Check sheet for the drawn part. Datum: minimum x, y, z corner. Units: mm. A direction names the side the tool comes from. Give positions to 0.01 mm unless a question says otherwise; leave off trailing zeros. Loops run counter-clockwise (first coordinate to the right, second up) from the corner with the lowest first, then second, coordinate; pieces in that order, holes last. Notation, with made-up numbers: (55, 76) - (111, 76) arc R5 ccw to (111, 81) - close; hole circle Ø11 at (3.5, 62.25). An arc over 180 degrees is marked (long way). One line per item, written item: value. Start each with the question number.
1. Sectioned sample at D-D (x = 14). Record the cut outline in (y, z), plus the area to 3 significant figures.
2. Scan lines: L1, parallel to X at y = 27, z = 47.5; L2, parallel to X at y = 30, z = 5; L3, parallel to X at y = 8, z = 27. Record each from-to range of solid material in increasing order. Write a range as [from, to].
3. Sectioned sample at A-A (y = 41.5). Record the cut outline in (x, z).
4. Access from +Z, -Z, +X, -X, +Y, -Y to the whole of each face (thin tool, end or side, straight path). Record for the marked faces 1, 2, 3 and 4.
5. Sectioned sample at B-B (z = 60). Count the separate pieces of the cut face and the enclosed holes in it, plus the area to 3 significant figures.
6. Gauge pin test, flat ends, axial feed: pin 1 (10 mm diameter, centred on x = 87.5, z = 50.5, fed in from +Y); pin 2 (1.5 mm diameter, centred on x = 72, y = 28, fed in from +Z); pin 3 (2 mm diameter, centred on x = 54, y = 32, fed in from +Z); pin 4 (8 mm diameter, centred on x = 96.5, z = 42, fed in from -Y). Record the tip position at first contact, or that the pin passes through.
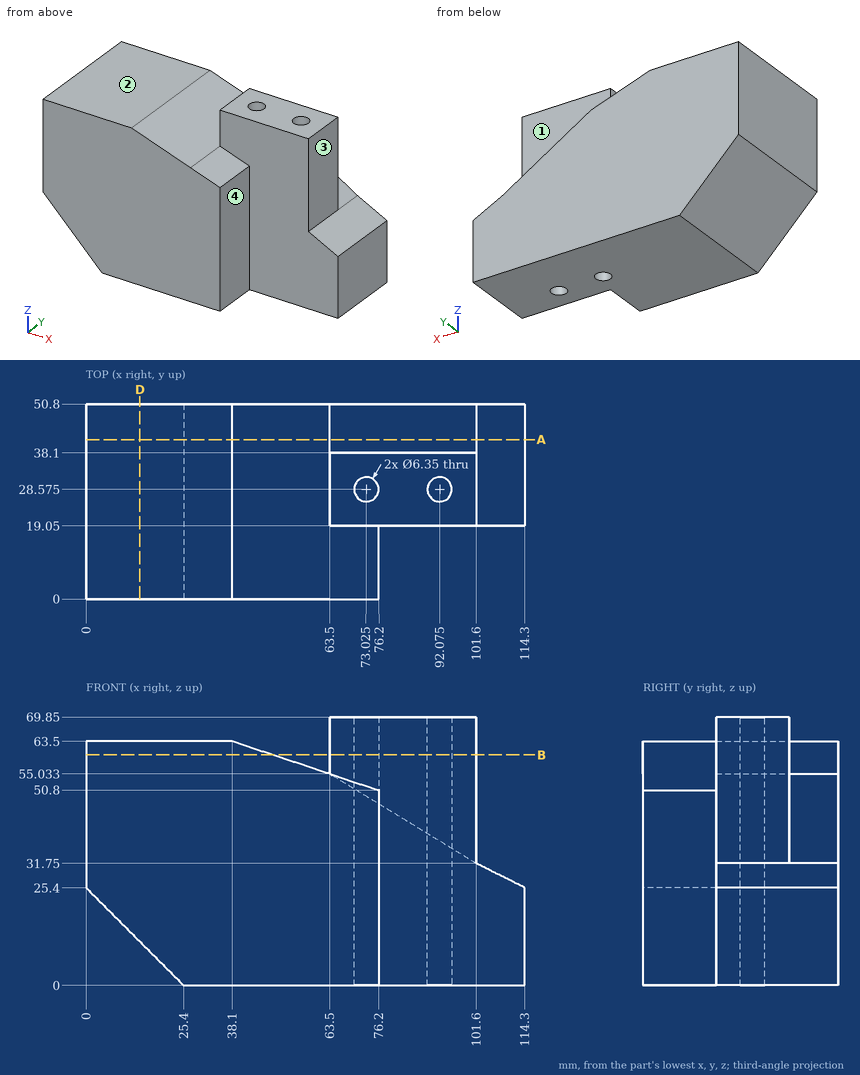
Results are:
1. outline: (0, 11.4) - (50.8, 11.4) - (50.8, 63.5) - (0, 63.5) - close
1. area: 2,650 mm^2
2. L1: x = [0, 70.27], [75.78, 89.32], [94.83, 101.6]
2. L2: x = [20.4, 70.19], [75.86, 89.24], [94.91, 114.3]
2. L3: x = [0, 76.2]
3. outline: (0, 25.4) - (25.4, 0) - (114.3, 0) - (114.3, 25.4) - (101.6, 31.75) - (63.5, 55.03) - (38.1, 63.5) - (0, 63.5) - close
4. face 1: +Z, +X, +Y
4. face 2: +Z, -X, +Y, -Y
4. face 3: +Z, +X, +Y, -Y
4. face 4: +Z, -Z, +X, -Y
5. separate pieces: 2
5. enclosed holes: 2
5. area: 3,130 mm^2
6. pin 1: stops at y = 38.1
6. pin 2: passes through
6. pin 3: stops at z = 58.53
6. pin 4: stops at y = 19.05
